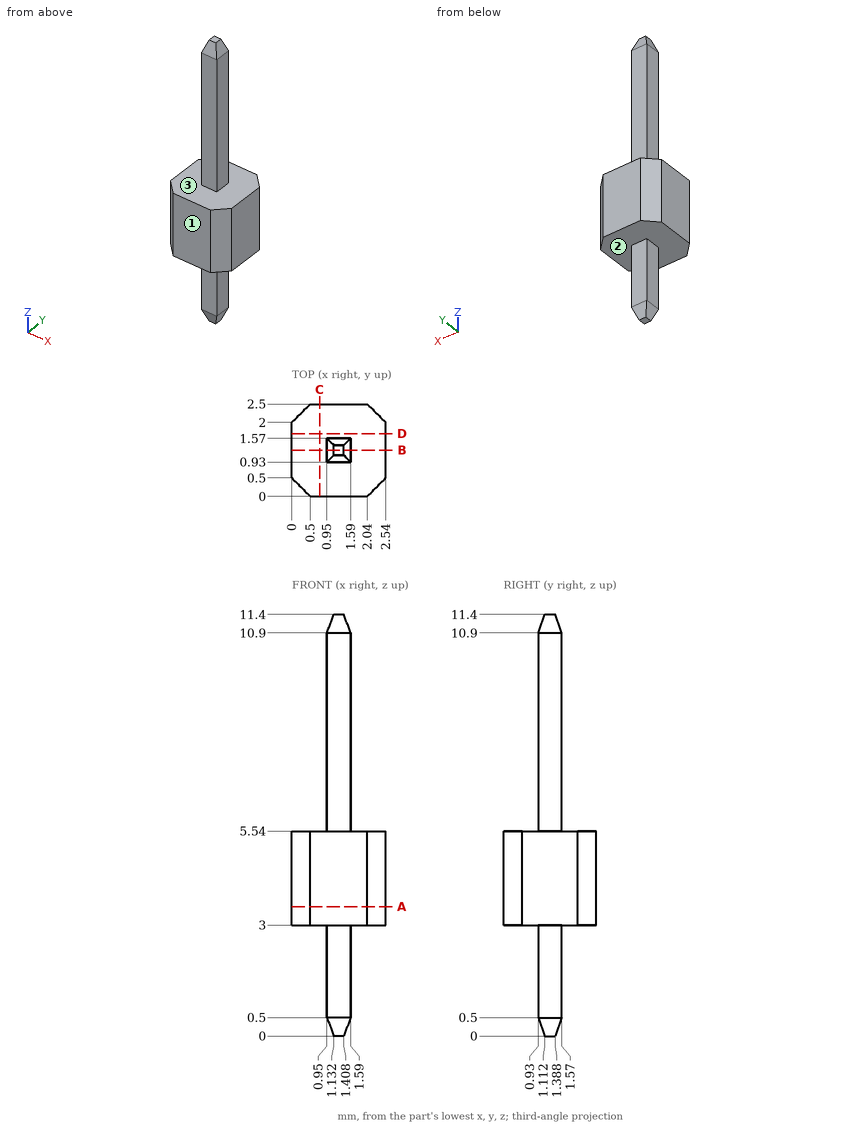
Drawing for the job (mm, zero at the part's lowest x, y, z). A direction names the side the tool comes from. Give positions to 0.01 mm unless a question says otherwise; leave off trailing zeros. Loops run counter-clockwise (first coordinate to the right, second up) from the corner with the lowest first, then second, coordinate; pieces in that order, holes last.
(1) Band-saw the part on A-A (z = 3.5). Write the cut outline in (x, y), and give its area (3 significant figures).
Return value:
outline: (0, 0.5) - (0.5, 0) - (2.04, 0) - (2.54, 0.5) - (2.54, 2) - (2.04, 2.5) - (0.5, 2.5) - (0, 2) - close
area: 5.85 mm2
(2) Band-saw the part on B-B (y = 1.25). Write the cut outline in (x, z), and give its area (3 significant figures).
Return value:
outline: (0, 3) - (0.95, 3) - (0.95, 0.5) - (1.13, 0) - (1.41, 0) - (1.59, 0.5) - (1.59, 3) - (2.54, 3) - (2.54, 5.54) - (1.59, 5.54) - (1.59, 10.9) - (1.41, 11.4) - (1.13, 11.4) - (0.95, 10.9) - (0.95, 5.54) - (0, 5.54) - close
area: 11.9 mm2
(3) Band-saw the part on C-C (x = 0.75). Write the cut outline in (y, z), and give its area (3 significant figures).
Return value:
outline: (0, 3) - (2.5, 3) - (2.5, 5.54) - (0, 5.54) - close
area: 6.35 mm2
(4) Band-saw the part on D-D (y = 1.7). Write the cut outline in (x, z).
Return value:
outline: (0, 3) - (2.54, 3) - (2.54, 5.54) - (0, 5.54) - close
(5) 3-axis set-ups, long thin cutter, end or side, ignore diameter. For the marked faces 1, 2 and 3: which of +Z, -Z, +X, -X, +Y, -Y reach the whole face in a straight line?
Return value:
face 1: +Z, -Z, +X, -X, -Y
face 2: -Z
face 3: +Z
(6) Drill centre lines: line 1 along X through (y, z) = (1.05, 6); line 2 along Y through (x, z) = (1.2, 8.75); line 3 along Z through (x, y) = (1.9, 1.5). Where is each one in solid material? Low to high.
Return value:
line 1: x = 0.95 to 1.59
line 2: y = 0.93 to 1.57
line 3: z = 3 to 5.54
(7) Pin check, flat tips, straight feed: pin 1 (1 mm diameter, centred on y = 1.5, z = 1.5, fed in from -X); pin 2 (0.5 mm diameter, centred on x = 1.5, z = 9, fed in from -Y); pin 3 (1 mm diameter, centred on x = 0.5, y = 2, fed in from +Z); pin 4 (1 mm diameter, centred on x = 0.5, z = 5.5, fed in from -Y). Stop position of each tip, or through.
Return value:
pin 1: stops at x = 0.95
pin 2: stops at y = 0.93
pin 3: stops at z = 5.54
pin 4: stops at y = 0
